Autodesk Inventor part; units mm, degrees
ref_plane "YZ Plane" through (0, 0, 0) normal (1, 0, 0) x (0, 1, 0)
ref_plane "XZ Plane" through (0, 0, 0) normal (0, 1, 0) x (-1, 0, 0)
ref_plane "XY Plane" through (0, 0, 0) normal (0, 0, 1) x (1, 0, 0)
sketch "草图1" plane through (0, 0, 0) normal (1, 0, 0) x (0, 1, 0)
  line L0 (3.6213, 2.1213) -> (1.5, 0)
  line L1 (1.5, 0) -> (-1.5, 0)
  line L2 (-1.5, 0) -> (-3.6213, 2.1213)
  line L3 (-3.6213, 2.1213) -> (-3.6213, 5.1213)
  line L4 (-3.6213, 5.1213) -> (-1.5, 7.2426)
  line L5 (-1.5, 7.2426) -> (1.5, 7.2426)
  line L6 (1.5, 7.2426) -> (3.6213, 5.1213)
  line L7 (3.6213, 5.1213) -> (3.6213, 2.1213)
  line L8 (1.608, 0) -> (-1.392, 0)
  line L9 (0, 0) -> (0, 9.8594)
  point P0 (0, 3.6213)
  dimension "d0" = 3
extrude "拉伸1" add sketch "草图1" along normal mid plane 10
sketch "草图2" plane through (-5, 0, 0) normal (-1, 0, 0) x (0, 0, 1)
  line L0 (2.1213, -3.6213) -> (5.1213, -3.6213)
  line L1 (5.1213, -3.6213) -> (7.2426, -1.5)
  line L2 (7.2426, -1.5) -> (7.2426, 1.5)
  line L3 (7.2426, 1.5) -> (5.1213, 3.6213)
  line L4 (5.1213, 3.6213) -> (2.1213, 3.6213)
  line L5 (2.1213, 3.6213) -> (0, 1.5)
  line L6 (0, 1.5) -> (0, -1.5)
  line L7 (0, -1.5) -> (2.1213, -3.6213)
  circle A0 centre (3.6213, 0) radius 1.5
  point P0 (0, 0)
  dimension "d3" = 3
hole "孔1" at (-5, 0, 3.6213) direction (1, 0, 0) diameter 3 end through all
properties part number "关节2"
Geometry check sheet. Reference: the model listing, model coordinates, mm. Give positions to 0.01 mm unless a question says otherwise; leave off trailing zeros. Order: outer loops, then holes, each group sorted by start corner. A loop starts at its lowest first (then second) coordinate and runs counter-clockwise, first axis right, second up.
1. Release check for a two-part mould opening along Y. For faces 1 (the face through (-0.07, -2.575, 6.167)), 2 (the face through (0.07, -0.066, 2.123)), 3 (the face through (0, 0, 0)) record: pulls with the +Y half, pulls with the -Y half, needs draft (parallel to the pull), parting line crosses it, or undercut.
2. Gauge pin test, flat end, axial feed: pin 1 Ø1 at (y, z) = (-1, 4) entering from +X. Record the tip position at first contact, or that the pin passes through.
3. Section check A-A, the plane y = 0. Enter the section's corners in (x, z).
4. Section check D-D, the plane z = 1.25. Enter the section's corners in (x, y).
5. Section check B-B, the plane x = -1.75. Enter the section's corners in (y, z).
6. Section check C-C, the plane z = 5. Enter the section's corners in (x, y).
7. Thickness scan on L1, parallel to Z at x = 1, y = 0; L2, parallel to Y at x = 2.75, z = 4.5; L3, parallel to Y at x = 2.25, z = 2.5. Record the ranges inside material, lowest first.
Values follow:
1. face 1: pulls with the -Y half
1. face 2: undercut
1. face 3: needs draft
2. pin 1: stops at x = 5
3. outline: (-5, 0) - (5, 0) - (5, 2.12) - (-5, 2.12) - close; (-5, 5.12) - (5, 5.12) - (5, 7.24) - (-5, 7.24) - close
4. outline: (-5, -2.75) - (5, -2.75) - (5, 2.75) - (-5, 2.75) - close
5. outline: (-3.62, 2.12) - (-1.5, 0) - (1.5, 0) - (3.62, 2.12) - (3.62, 5.12) - (1.5, 7.24) - (-1.5, 7.24) - (-3.62, 5.12) - close; hole circle Ø3 at (0, 3.62)
6. outline: (-5, -3.62) - (5, -3.62) - (5, -0.59) - (-5, -0.59) - close; (-5, 0.59) - (5, 0.59) - (5, 3.62) - (-5, 3.62) - close
7. L1: z = 0 to 2.12, 5.12 to 7.24
7. L2: y = -3.62 to -1.22, 1.22 to 3.62
7. L3: y = -3.62 to -1, 1 to 3.62
